Geometry check sheet. Reference: the model listing, model coordinates, mm. Face numbers are marked on the shaded views. Coordinates: 2 decimals unless noted, no trailing zeros. Write each loop counter-clockwise with the first axis right and the second up, starting at its lowest first coordinate (ties: lowest second). Pieces come first, ordered by that corner, then holes. Notation, with made-up numbers: M 55.25,-12.75 L 92.25,-12.75 A18 cw 92.25,-7.75 Z; hole C -16.75,-6 d6. An arc over 180 degrees is marked long. Answer as a JSON object with one key per item and string values. Group by question number.
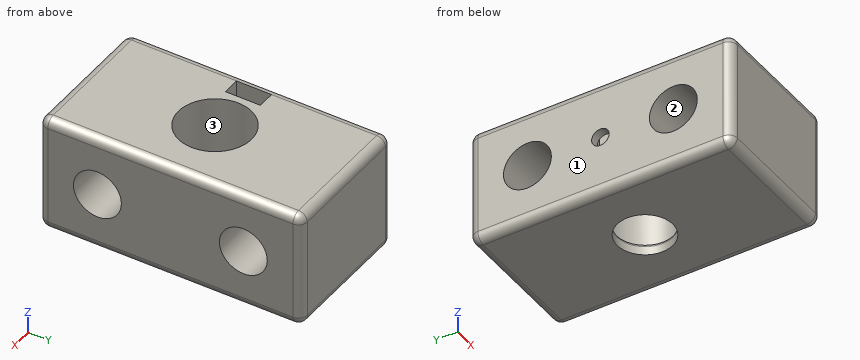
```python
from build123d import *

# Parameters (mm, degrees)
SKETCH1_W      = 24
SKETCH1_H      = 45
EXTRUDE1_DEPTH = 20
SKETCH2_R      = 4.1
EXTRUDE2_DEPTH = 39.5
SKETCH3_R      = 6.25
EXTRUDE3_DEPTH = 18
SKETCH4_R      = 4.75
EXTRUDE4_DEPTH = 18
SKETCH5_W      = 3
SKETCH5_H      = 6
EXTRUDE5_DEPTH = 14
SKETCH6_R      = 1.5
EXTRUDE6_DEPTH = 13
FILLET1_R      = 1.5
FILLET2_R      = 0.5
FILLET3_R      = 3


with BuildPart() as part:
    # Sketch1 → Extrude1 (new body)
    with BuildSketch(Plane.XY):
        Rectangle(SKETCH1_W, SKETCH1_H)
    extrude(amount=EXTRUDE1_DEPTH)

    # Sketch2 → Extrude2 (cut, through all)
    with BuildSketch(Plane(origin=(12, 0, 0), x_dir=(0, 0, -1), z_dir=(1, 0, 0))):
        with Locations((-10, 12.5)):
            Circle(SKETCH2_R)
        with Locations(Location((-10, -12.5, 0), (0, 0, 180))):
            Circle(SKETCH2_R)
    extrude(amount=-EXTRUDE2_DEPTH, mode=Mode.SUBTRACT)

    # Sketch3 → Extrude3 (cut)
    with BuildSketch(Plane.XY.offset(20)):
        Circle(SKETCH3_R)
    extrude(amount=-EXTRUDE3_DEPTH, mode=Mode.SUBTRACT)

    # Sketch4 → Extrude4 (cut)
    with BuildSketch(Plane.XY.offset(2)):
        Circle(SKETCH4_R)
    extrude(amount=-EXTRUDE4_DEPTH, mode=Mode.SUBTRACT)

    # Sketch5 → Extrude5 (cut)
    with BuildSketch(Plane.XY.offset(20)):
        with Locations((-9, 0)):
            Rectangle(SKETCH5_W, SKETCH5_H)
    extrude(amount=-EXTRUDE5_DEPTH, mode=Mode.SUBTRACT)

    # Sketch6 → Extrude6 (cut)
    with BuildSketch(Plane.ZY.offset(12)):
        with Locations((10, 0)):
            Circle(SKETCH6_R)
    extrude(amount=-EXTRUDE6_DEPTH, mode=Mode.SUBTRACT)

    # Fillet1
    fillet1_edges = [part.edges().sort_by_distance(p)[0] for p in [
        (12, 0, 20),
        (0, 22.5, 20),
        (-12, 0, 20),
        (0, 22.5, 0),
        (12, 0, 0),
        (0, -22.5, 0),
        (-12, 0, 0),
        (0, -22.5, 20),
        (-12, 22.5, 10),
        (12, 22.5, 10),
        (12, -22.5, 10),
        (-12, -22.5, 10),
    ]]
    fillet(fillet1_edges, radius=FILLET1_R - 0.0001)  # a hair under: the kernel refuses the full size

    # Fillet2
    fillet2_edges = [part.edges().sort_by_distance(p)[0] for p in [
        (-4.75, 0, 2),
    ]]
    fillet(fillet2_edges, radius=FILLET2_R)

    # Fillet3
    fillet3_edges = [part.edges().sort_by_distance(p)[0] for p in [
        (-9, -3, 6),
        (-9, 3, 6),
    ]]
    fillet(fillet3_edges, radius=FILLET3_R - 0.0001)  # a hair under: the kernel refuses the full size


solid = part.part
```
1) Section check A-A (x = 0). Record the cut outline in (y, z), then the cut area to 3 significant figures.
2) Go/stop test with flat-tipped pins: pin 1 Ø1.8 at (y, z) = (0, 10) entering from -X; pin 2 Ø5 at (y, z) = (-12.5, 10) entering from -X; pin 3 Ø2.5 at (y, z) = (0, 10) entering from -X; pin 4 Ø11 at (x, y) = (0, 0) entering from +Z. Record where each tip stops, or that it passes through.
3) Material ranges on probe 1 along Y at (x, z) = (-6.7, 10); probe 2 along Y at (x, z) = (-8, 6.75); probe 3 along Y at (x, z) = (10, 12), recorded low to high. Write a range as [from, to].
4) Draft check along X on the marked faces 1, 2 and 3. Enter one of: +X half, -X half, draft (parallel to the pull), parting line (faces both ways), or undercut.
5) Section check B-B (y = 12.5). Record the cut outline in (x, z).
6) Section check D-D (x = -8.75). State how many separate pieces and enclosed holes the cut face has, then the cut area to 3 significant figures.
7) Section check C-C (z = 10). Record the cut outline in (x, y).
Entries:
{
 "1": {"outline": "M -22.5,1.5 A1.5 ccw -21,0 L -4.75,0 L -4.75,1.5 A0.5 ccw -5.25,2 L -6.25,2 L -6.25,20 L -21,20 A1.5 ccw -22.5,18.5 Z; M 4.75,0 L 21,0 A1.5 ccw 22.5,1.5 L 22.5,18.5 A1.5 ccw 21,20 L 6.25,20 L 6.25,2 L 5.25,2 A0.5 ccw 4.75,1.5 Z; hole C -12.5,10 d8.2; hole C 12.5,10 d8.2", "area": "548 mm^2"},
 "2": {"pin 1": "x = 6.18", "pin 2": "through", "pin 3": "x = 6.12", "pin 4": "z = 2"},
 "3": {"probe 1": "[-22.5, -16.6], [-8.4, -1.5], [1.5, 8.4], [16.6, 22.5]", "probe 2": "[-22.5, -15], [-10, -1.98], [1.98, 10], [15, 22.5]", "probe 3": "[-22.5, -16.08], [-8.92, 8.92], [16.08, 22.5]"},
 "4": {"face 1": "-X half", "face 2": "draft", "face 3": "undercut"},
 "5": {"outline": "M -12,1.5 A1.5 ccw -10.5,0 L 10.5,0 A1.5 ccw 12,1.5 L 12,5.9 L -12,5.9 Z; M -12,14.1 L 12,14.1 L 12,18.5 A1.5 ccw 10.5,20 L -10.5,20 A1.5 ccw -12,18.5 Z"},
 "6": {"separate pieces": "1", "enclosed holes": "2", "area": "712 mm^2"},
 "7": {"outline": "M -12,-21 A1.5 ccw -10.5,-22.5 L 10.5,-22.5 A1.5 ccw 12,-21 L 12,-16.6 L -12,-16.6 Z; M -12,-8.4 L 12,-8.4 L 12,8.4 L -12,8.4 L -12,1.5 L -10.5,1.5 L -10.5,3 L -7.5,3 L -7.5,1.5 L -6.07,1.5 A6.25 cw long -6.07,-1.5 L -7.5,-1.5 L -7.5,-3 L -10.5,-3 L -10.5,-1.5 L -12,-1.5 Z; M -12,16.6 L 12,16.6 L 12,21 A1.5 ccw 10.5,22.5 L -10.5,22.5 A1.5 ccw -12,21 Z"}
}
